Verification items for the finished model (mm, model axes). Coordinates: 2 decimals unless noted, no trailing zeros. Write each loop counter-clockwise with the first axis right and the second up, starting at its lowest first coordinate (ties: lowest second). Pieces come first, ordered by that corner, then holes. Notation, with made-up numbers: M -20.75,16 L 20.25,16 A27 ccw 20.25,32 Z; hole C 15.25,11 d5. An arc over 180 degrees is marked long. Answer in a Markdown table with one row per item.
from build123d import *

# Parameters (mm, degrees)
SKETCH030_AS_DRAWN_R                      = 5
EXTRUDE025_DEPTH                          = 25.4
EXTRUDE025_ONTO_SKETCH030_PLACEMENT_ANGLE = 8
SKETCH018_AS_DRAWN_R                      = 1.2
EXTRUDE009_DEPTH                          = 7.8
EXTRUDE009_ONTO_SKETCH018_PLACEMENT_ANGLE = 8
EXTRUDE010_DEPTH                          = 1.4
EXTRUDE010_ONTO_SKETCH019_PLACEMENT_ANGLE = 8


with BuildPart() as plate_led_holes:
    # Sketch030 as drawn → Extrude025 (new, symmetric)
    with BuildSketch(Plane.XY):
        with Locations((78.81499, 41.5191)):
            Circle(SKETCH030_AS_DRAWN_R)
        with Locations((97.448702, 45.479818)):
            Circle(SKETCH030_AS_DRAWN_R)
        with Locations((116.082414, 49.440535)):
            Circle(SKETCH030_AS_DRAWN_R)
    extrude(amount=EXTRUDE025_DEPTH, both=True)


with BuildPart() as plate_led_holes_1:
    # Extrude025 onto Sketch030 placement: moved
    add(plate_led_holes.part.moved(Location((42.3672, 0, 47.625))).rotate(Axis((42.3672, 0, 47.625), (0, 1, 0)), EXTRUDE025_ONTO_SKETCH030_PLACEMENT_ANGLE))


with BuildPart() as screw_hole_cuts:
    # Sketch018 as drawn → Extrude009 (new)
    with BuildSketch(Plane.XY):
        with Locations((-31.998318, 84.649891)):
            Circle(SKETCH018_AS_DRAWN_R)
        with Locations((-31.998318, -89.695043)):
            Circle(SKETCH018_AS_DRAWN_R)
        with Locations((156.654735, -49.595599)):
            Circle(SKETCH018_AS_DRAWN_R)
        with Locations((156.654735, 84.649891)):
            Circle(SKETCH018_AS_DRAWN_R)
    extrude(amount=EXTRUDE009_DEPTH)


with BuildPart() as screw_hole_cuts_1:
    # Extrude009 onto Sketch018 placement: moved
    add(screw_hole_cuts.part.moved(Location((39.98734, 0, 30.691416))).rotate(Axis((39.98734, 0, 30.691416), (0, 1, 0)), EXTRUDE009_ONTO_SKETCH018_PLACEMENT_ANGLE))


with BuildPart() as cut017:
    # Sketch019 as drawn → Extrude010 (new)
    with BuildSketch(Plane.XY):
        with BuildLine():
            Line((-37.205318, 86.681891), (-37.205318, -92.017095))
            ThreePointArc((-37.205318, -92.017095), (-36.028411, -94.484534), (-33.370199, -95.122714))
            Line((-33.370199, -95.122714), (159.34685, -54.159441))
            ThreePointArc((159.34685, -54.159441), (161.154172, -53.051915), (161.861735, -51.053821))
            Line((161.861735, -51.053821), (161.861735, 86.681892))
            ThreePointArc((161.861735, 86.681892), (160.931799, 88.926956), (158.686734, 89.856891))
            Line((158.686734, 89.856891), (-34.030318, 89.856891))
            ThreePointArc((-34.030318, 89.856891), (-36.275382, 88.926955), (-37.205318, 86.681891))
        make_face()
    extrude(amount=EXTRUDE010_DEPTH)


with BuildPart() as cut017_1:
    # Extrude010 onto Sketch019 placement: moved
    add(cut017.part.moved(Location((39.98734, 0, 30.691416))).rotate(Axis((39.98734, 0, 30.691416), (0, 1, 0)), EXTRUDE010_ONTO_SKETCH019_PLACEMENT_ANGLE))

    # Cut002: cut Screw Hole Cuts
    add(screw_hole_cuts_1.part, mode=Mode.SUBTRACT)

    # Cut017: cut Plate LED Holes
    add(plate_led_holes_1.part, mode=Mode.SUBTRACT)


solid = cut017_1.part
1) Sectioned sample at A-A (y = 63.5). Record the cut outline in (x, z).
Response values:
| item | result |
|---|---|
| outline | M 3.14,35.87 L 200.27,8.16 L 200.47,9.55 L 3.34,37.26 Z |
2) Depth check by flat-ended pin: pin 1 (12 mm diameter, centred on x = 26, z = 23, fed in from +Y); pin 2 (5 mm diameter, centred on x = 90.5, y = 28, fed in from +Z); pin 3 (4 mm diameter, centred on x = 39.5, y = 28, fed in from +Z); pin 4 (4 mm diameter, centred on x = 51, y = -74, fed in from -Z). Enter the tip coordinate at first touch or a pass-through.
Response values:
| item | result |
|---|---|
| pin 1 | passes through |
| pin 2 | stops at z = 25.36 |
| pin 3 | stops at z = 32.45 |
| pin 4 | stops at z = 28.86 |
3) Thickness scan on L1, parallel to Z at x = 85, y = -60.5; L2, parallel to Z at x = 183, y = 3; L3, parallel to Y at x = 106, z = 22. Record the ranges inside material, lowest first. Write a range as [from, to].
Response values:
| item | result |
|---|---|
| L1 | z = [24.37, 25.78] |
| L2 | z = [10.59, 12.01] |
| L3 | y = [-73.88, 89.86] |
4) Sectioned sample at B-B (z = 31.5). Record the cut outline in (x, y).
Response values:
| item | result |
|---|---|
| outline | M 34.23,-89.26 L 44.29,-87.15 L 44.29,89.86 L 34.23,89.86 Z |
5) Release check for a two-part mould opening along Y. For faces 1 (the face through (154.4, 54.4, 15.3)), 2 (the face through (103, 89.857, 23)), 3 (the face through (100.5, -1.4, 23.6)), 4 (the face through (114.485, 44.898, 20.938)) record: +Y half, -Y half, draft (parallel to the pull), parting line (faces both ways), or undercut.
Response values:
| item | result |
|---|---|
| face 1 | undercut |
| face 2 | +Y half |
| face 3 | draft |
| face 4 | undercut |
